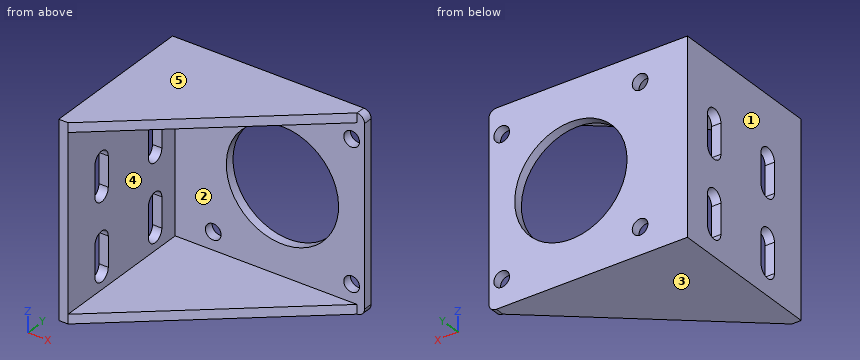
```python
from build123d import *

# Parameters (mm, degrees)
SKETCH1_W           = 67.6275
SKETCH1_H           = 65.405
SKETCH1_R           = 19.1135
SKETCH1_R_2         = 2.667
BOSS_EXTRUDE1_DEPTH = 3.175
FILLET1_R           = 2.54
SKETCH2_W           = 65.405
SKETCH2_H           = 50.8
BOSS_EXTRUDE2_DEPTH = 3.175
BOSS_EXTRUDE5_DEPTH = 3.175
BOSS_EXTRUDE6_DEPTH = 3.175
SKETCH9_R           = 3.175
CUT_EXTRUDE1_DEPTH  = 3.175


with BuildPart() as part:
    # Sketch1 → Boss-Extrude1 (new body)
    with BuildSketch(Plane(origin=(0, 0, 0), x_dir=(1, 0, 0), z_dir=(0, 1, 0))):
        with Locations((-5.87375, 0)):
            Rectangle(SKETCH1_W, SKETCH1_H)
        with Locations(Location((0, 0, 0), (0, 0, 270))):
            Circle(SKETCH1_R, mode=Mode.SUBTRACT)
        with Locations(Location((-23.5585, 23.5585, 0), (0, 0, 270))):
            Circle(SKETCH1_R_2, mode=Mode.SUBTRACT)
        with Locations(Location((23.5585, 23.5585, 0), (0, 0, 270))):
            Circle(SKETCH1_R_2, mode=Mode.SUBTRACT)
        with Locations(Location((-23.5585, -23.5585, 0), (0, 0, 270))):
            Circle(SKETCH1_R_2, mode=Mode.SUBTRACT)
        with Locations(Location((23.5585, -23.5585, 0), (0, 0, 270))):
            Circle(SKETCH1_R_2, mode=Mode.SUBTRACT)
    extrude(amount=BOSS_EXTRUDE1_DEPTH)

    # Fillet1
    fillet1_edges = [part.edges().sort_by_distance(p)[0] for p in [
        (27.94, 1.5875, -32.7025),
        (27.94, 1.5875, 32.7025),
    ]]
    fillet(fillet1_edges, radius=FILLET1_R)

    # Sketch2 → Boss-Extrude2 (add)
    with BuildSketch(Plane.ZY.offset(39.6875)):
        with Locations((0, -25.4)):
            Rectangle(SKETCH2_W, SKETCH2_H)
    extrude(amount=-BOSS_EXTRUDE2_DEPTH)

    # Sketch7 → Boss-Extrude5 (add)
    with BuildSketch(Plane.XY.offset(32.7025)):
        Polygon((-36.5125, -50.8), (25.4, 0), (-36.5125, 0), align=None)
    extrude(amount=-BOSS_EXTRUDE5_DEPTH)

    # Sketch8 → Boss-Extrude6 (add)
    with BuildSketch(Plane(origin=(0, 0, -32.7025), x_dir=(-1, 0, 0), z_dir=(0, 0, -1))):
        Polygon((-25.4, 0), (36.5125, 0), (36.5125, -50.8), align=None)
    extrude(amount=-BOSS_EXTRUDE6_DEPTH)

    # Sketch9 → Cut-Extrude1 (cut)
    with BuildSketch(Plane(origin=(-36.5125, 0, 0), x_dir=(0, 0, -1), z_dir=(1, 0, 0))):
        with BuildLine():
            ThreePointArc((-2.2225, -12.7), (-5.3975, -9.525), (-2.2225, -6.35))
            Line((-2.2225, -6.35), (-12.3825, -6.35))
            ThreePointArc((-12.3825, -6.35), (-10.13743597, -7.27993597), (-9.2075, -9.525))
            ThreePointArc((-9.2075, -9.525), (-10.13743597, -11.77006403), (-12.3825, -12.7))
            Line((-12.3825, -12.7), (-2.2225, -12.7))
        make_face()
        with Locations((-2.2225, -9.525)):
            Circle(SKETCH9_R)
        with Locations((-12.3825, -9.525)):
            Circle(SKETCH9_R)
        with BuildLine():
            ThreePointArc((23.8125, -12.7), (20.6375, -9.525), (23.8125, -6.35))
            Line((23.8125, -6.35), (13.6525, -6.35))
            ThreePointArc((13.6525, -6.35), (15.89756403, -7.27993597), (16.8275, -9.525))
            ThreePointArc((16.8275, -9.525), (15.89756403, -11.77006403), (13.6525, -12.7))
            Line((13.6525, -12.7), (23.8125, -12.7))
        make_face()
        with Locations((13.6525, -9.525)):
            Circle(SKETCH9_R)
        with Locations((23.8125, -9.525)):
            Circle(SKETCH9_R)
        with Locations((23.8125, -34.925)):
            Circle(SKETCH9_R)
        with BuildLine():
            Line((13.6525, -38.1), (23.8125, -38.1))
            ThreePointArc((23.8125, -38.1), (20.6375, -34.925), (23.8125, -31.75))
            Line((23.8125, -31.75), (13.6525, -31.75))
            ThreePointArc((13.6525, -31.75), (15.89756403, -32.67993597), (16.8275, -34.925))
            ThreePointArc((16.8275, -34.925), (15.89756403, -37.17006403), (13.6525, -38.1))
        make_face()
        with Locations((13.6525, -34.925)):
            Circle(SKETCH9_R)
        with Locations((-2.2225, -34.925)):
            Circle(SKETCH9_R)
        with BuildLine():
            ThreePointArc((-2.2225, -38.1), (-5.3975, -34.925), (-2.2225, -31.75))
            Line((-2.2225, -31.75), (-12.3825, -31.75))
            ThreePointArc((-12.3825, -31.75), (-10.13743597, -32.67993597), (-9.2075, -34.925))
            ThreePointArc((-9.2075, -34.925), (-10.13743597, -37.17006403), (-12.3825, -38.1))
            Line((-12.3825, -38.1), (-2.2225, -38.1))
        make_face()
        with Locations((-12.3825, -34.925)):
            Circle(SKETCH9_R)
    extrude(amount=-CUT_EXTRUDE1_DEPTH, mode=Mode.SUBTRACT)


solid = part.part
```
Input: part model. Units: mm. Frame: model coordinates. Face numbers are marked on the shaded views. A direction names the side the tool comes from. Give positions to 0.01 mm unless a question says otherwise; leave off trailing zeros. Order: outer loops, then holes, each group sorted by start corner. A loop starts at its lowest first (then second) coordinate and runs counter-clockwise, first axis right, second up.
1. Cut plane D-D (x = 7). Return loops of the section in (y, z) (1 decimal).
Computed:
outline: (-15.1, -32.7) - (3.2, -32.7) - (3.2, -17.8) - (0, -17.8) - (0, -29.5) - (-15.1, -29.5) - close; (-15.1, 29.5) - (0, 29.5) - (0, 17.8) - (3.2, 17.8) - (3.2, 32.7) - (-15.1, 32.7) - close
2. Cut plane A-A (z = -20). State how many separate pieces and enclosed holes the cut face has, and give its area (3 significant figures).
Computed:
separate pieces: 3
enclosed holes: 0
area: 336 mm2
3. Draft query along Z for the marked faces 3, 4 and 5. Return one class per face: released by +Z, released by -Z, zero draft, split by the parting line, or undercut.
Computed:
face 3: released by -Z
face 4: undercut
face 5: released by +Z
4. Line query: probe 1 along X at (y, z) = (2, 0); probe 2 along Z at (x, y) = (-6, -4); probe 3 along X at (y, z) = (-43, 29). Output: solid intervals per line, ascending.
Computed:
probe 1: x = -39.69 to -19.11, 19.11 to 27.94
probe 2: z = -32.7 to -29.53, 29.53 to 32.7
probe 3: x = -39.69 to -36.51
5. Pin query (flat end, axial travel): pin 1 Ø4 at (y, z) = (-22, -2) entering from +X; pin 2 Ø8 at (x, z) = (-18.5, 1) entering from +Y (3 decimals). Return the tip coordinate at first contact, or that it passes through.
Computed:
pin 1: stops at x = -36.51
pin 2: stops at y = 3.175
6. Cut plane C-C (y = -24). Return loops of the section in (x, z), and give its area (3 significant figures).
Computed:
outline: (-39.69, -32.7) - (-3.85, -32.7) - (-3.85, -29.53) - (-36.51, -29.53) - (-36.51, 29.53) - (-3.85, 29.53) - (-3.85, 32.7) - (-39.69, 32.7) - close
area: 415 mm2
7. Cut plane B-B (x = 22.5). Return loops of the section in (y, z) (1 decimal), and give its area (3 significant figures).
Computed:
outline: (-2.4, -32.7) - (3.2, -32.7) - (3.2, -26) - (0, -26) - (0, -29.5) - (-2.4, -29.5) - close; (-2.4, 29.5) - (0, 29.5) - (0, 26) - (3.2, 26) - (3.2, 32.7) - (-2.4, 32.7) - close; (0, -21.1) - (3.2, -21.1) - (3.2, 21.1) - (0, 21.1) - close
area: 192 mm2
8. Set-up query: the marked faces 1 and 2. Return all of +Z, -Z, +X, -X, +Y, -Y with unobstructed straight access to the full face (end or side cutting, diameter ignored); none if empty.
Computed:
face 1: +Z, -Z, -X, +Y, -Y
face 2: +X, -Y
